Build history of the part. All positions in model axes, mm. A direction names the side the tool comes from. Give positions to 0.01 mm unless a question says otherwise; leave off trailing zeros. Loops run counter-clockwise (first coordinate to the right, second up) from the corner with the lowest first, then second, coordinate; pieces in that order, holes last. Notation, with made-up numbers: (9.5, -6.5) -> (37.5, -6.5) arc R8 cw to (37.5, 4.5) -> close; hole circle Ø10 at (8.25, -19.75). An arc over 180 degrees is marked (long way). Answer as a JSON object with one key per item and string values. Group by question number.
Q1. Drop flat-ended pins along their axis: pin 1 (5.5 mm diameter, centred on x = 16.5, y = -5, fed in from +Z); pin 2 (3.5 mm diameter, centred on x = 62.95, y = 24.95, fed in from -Z); pin 3 (5.5 mm diameter, centred on x = -15, y = -6, fed in from -Z); pin 4 (4 mm diameter, centred on y = -16, z = 15.5, fed in from +X). Give the stop position or say it passes through.
Q2. Wall check: probe 1 along Y at (x, z) = (-5, 31.5) (3 decimals); probe 2 along Y at (x, z) = (-62.95, 1.55); probe 3 along X at (y, z) = (4, 22). Give the ranges that are in metal, low to high. Write a range as from..to.
Q3. Band-saw the part on C-C, the plane z = 24.5. Write the cut outline in (x, y), plus the area to 3 significant figures.
Q4. Tool access for faces 4 (the flat face through (-63, 0, 2)), 5 (the flat face through (-56.217, 0.49, 1.38)), 6 (the cylindrical face through (27.379, -26.486, 31.186)), 7 (the cylindrical face through (-64.9, -25, 1)): list every direction of +Z, -Z, +X, -X, +Y, -Y with a clear straight run to the whole face (end or side of a thin tool).
Q5. Band-saw the part on D-D, the plane x = -50. Write the cut outline in (y, z).
Q6. Band-saw the part on A-A, the plane y = -6. Write the cut outline in (x, z), plus the area to 3 significant figures.
Q7. Band-saw the part on B-B, the plane x = 5. Write the cut outline in (y, z) (3 decimals), plus the area to 3 significant figures.
Q8. Two-plate mould, pull along X, no slides. Class faces 1 (the flat face through (49.64, -23.56, 31.01)), 2 (the flat face through (1, 27, 27.6)), 3 (the cylindrical face through (-11.767, -7.341, 27.354)): pulls with the +X half, pulls with the -X half, needs draft (parallel to the pull), parting line crosses it, or undercut.
from build123d import *

# Parameters (mm, degrees)
F0_W      = 132
F0_H      = 70
F1_DEPTH  = 2
F3_DEPTH  = 35
F4_DEPTH  = 35
F6_DEPTH  = 23.2
F7_R      = 1.95
F8_DEPTH  = 25
F9_R      = 3
F10_R     = 2.575
F11_DEPTH = 5.2
F13_DEPTH = 70.001
F14_W     = 35
F14_H     = 25
F14_R     = 3.5
F14_W_2   = 14.5
F14_H_2   = 15
F15_DEPTH = 0.5


with BuildPart() as f1:
    # F0 (on Top) → F1 (new body)
    with BuildSketch(Plane.XY):
        Rectangle(F0_W, F0_H)
    extrude(amount=F1_DEPTH)

    # F2 (on Front) → F3 (join, through all)
    with BuildSketch(Plane.XZ):
        Polygon((-52.3, 14.7), (-59.5, 2), (59.5, 2), (52.3, 14.7), (52.3, 22.2), (46.9, 27.6), (-46.9, 27.6), (-52.3, 22.2), align=None)
    extrude(amount=F3_DEPTH)

    # F2 (on Front) → F4 (join, through all)
    with BuildSketch(Plane.XZ):
        Polygon((-52.3, 14.7), (-59.5, 2), (59.5, 2), (52.3, 14.7), (52.3, 22.2), (46.9, 27.6), (-46.9, 27.6), (-52.3, 22.2), align=None)
    extrude(amount=-F4_DEPTH)

    # F5 (on face) → F6 (join)
    with BuildSketch(Plane.XZ.offset(35)):
        Polygon((-52.3, 28.35), (-52.3, 22.2), (-46.9, 27.6), (46.9, 27.6), (52.3, 22.2), (52.3, 28.35), (46.9, 33.75), (-46.9, 33.75), align=None)
    extrude(amount=-F6_DEPTH)

    # F7 (on face) → F8 (cut)
    with BuildSketch(Plane(origin=(0, 0, 0), x_dir=(1, 0, 0), z_dir=(0, 0, -1))):
        with Locations((62.95, -24.95)):
            Circle(F7_R)
        with Locations((62.95, 24.95)):
            Circle(F7_R)
        with Locations((-62.95, 24.95)):
            Circle(F7_R)
        with Locations((-62.95, -24.95)):
            Circle(F7_R)
    extrude(amount=-F8_DEPTH, mode=Mode.SUBTRACT)

    # F9
    f9_edges = [f1.edges().sort_by_distance(p)[0] for p in [
        (66, -35, 1),
        (66, 35, 1),
        (-66, -35, 1),
        (-66, 35, 1),
    ]]
    fillet(f9_edges, radius=F9_R)

    # F10 (on face) → F11 (cut)
    with BuildSketch(Plane.XY.offset(33.75)):
        with Locations((-25, -25.5)):
            Circle(F10_R)
        with Locations((-15, -25.5)):
            Circle(F10_R)
        with Locations((-5, -25.5)):
            Circle(F10_R)
        with Locations((5, -25.5)):
            Circle(F10_R)
        with Locations((15, -25.5)):
            Circle(F10_R)
        with Locations((25, -25.5)):
            Circle(F10_R)
    extrude(amount=-F11_DEPTH, mode=Mode.SUBTRACT)

    # F12 (on face) → F13 (cut, through all)
    with BuildSketch(Plane(origin=(0, 35, 0), x_dir=(-1, 0, 0), z_dir=(0, 1, 0))):
        Polygon((-57, 0), (57, 0), (55.412598, 2.8), (-55.412598, 2.8), align=None)
    extrude(amount=-F13_DEPTH, mode=Mode.SUBTRACT)

    # F14 (on face) → F15 (cut)
    with BuildSketch(Plane.XY.offset(27.6)):
        with Locations((0, 12.5)):
            Rectangle(F14_W, F14_H)
        with Locations((0, -6)):
            Circle(F14_R)
        with Locations((-15, -6)):
            Circle(F14_R)
        with Locations((15, -6)):
            Circle(F14_R)
        with Locations((36, 17.5)):
            Rectangle(F14_W_2, F14_H_2)
    extrude(amount=-F15_DEPTH, mode=Mode.SUBTRACT)


solid = f1.part
Worked answers:
{
 "1": {"pin 1": "z = 27.6", "pin 2": "through", "pin 3": "z = 2.8", "pin 4": "x = 52.98"},
 "2": {"probe 1": "-35..-28.075, -22.925..-11.8", "probe 2": "-35..-26.9, -23..23, 26.9..35", "probe 3": "-52.3..52.3"},
 "3": {"outline": "(-52.3, -35) -> (52.3, -35) -> (52.3, -11.8) -> (50, -11.8) -> (50, 35) -> (-50, 35) -> (-50, -11.8) -> (-52.3, -11.8) -> close", "area": "7,110 mm2"},
 "4": {"face 4": "+Z, -X, +Y, -Y", "face 5": "-Z, +Y, -Y", "face 6": "+Z", "face 7": "+Z, -Z"},
 "5": {"outline": "(-35, 2.8) -> (35, 2.8) -> (35, 24.5) -> (-11.8, 24.5) -> (-11.8, 30.65) -> (-35, 30.65) -> close"},
 "6": {"outline": "(-66, 0) -> (-57, 0) -> (-55.41, 2.8) -> (55.41, 2.8) -> (57, 0) -> (66, 0) -> (66, 2) -> (59.5, 2) -> (52.3, 14.7) -> (52.3, 22.2) -> (46.9, 27.6) -> (18.5, 27.6) -> (18.5, 27.1) -> (11.5, 27.1) -> (11.5, 27.6) -> (3.5, 27.6) -> (3.5, 27.1) -> (-3.5, 27.1) -> (-3.5, 27.6) -> (-11.5, 27.6) -> (-11.5, 27.1) -> (-18.5, 27.1) -> (-18.5, 27.6) -> (-46.9, 27.6) -> (-52.3, 22.2) -> (-52.3, 14.7) -> (-59.5, 2) -> (-66, 2) -> close", "area": "2,680 mm2"},
 "7": {"outline": "(-35, 2.8) -> (35, 2.8) -> (35, 27.6) -> (25, 27.6) -> (25, 27.1) -> (0, 27.1) -> (0, 27.6) -> (-11.8, 27.6) -> (-11.8, 33.75) -> (-22.925, 33.75) -> (-22.925, 28.55) -> (-28.075, 28.55) -> (-28.075, 33.75) -> (-35, 33.75) -> close", "area": "1,840 mm2"},
 "8": {"face 1": "pulls with the +X half", "face 2": "needs draft", "face 3": "undercut"}
}
